Drawing for the job (mm, zero at the part's lowest x, y, z). Give positions to 0.01 mm unless a question says otherwise; leave off trailing zeros. Loops run counter-clockwise (first coordinate to the right, second up) from the corner with the lowest first, then second, coordinate; pieces in that order, holes last. Notation, with made-up numbers: (-11.75, 61) -> (10.25, 61) arc R20 ccw to (10.25, 74) -> close; hole circle Ø3 at (9.5, 86). An arc over 180 degrees is marked (long way). Write item = value, one per line.
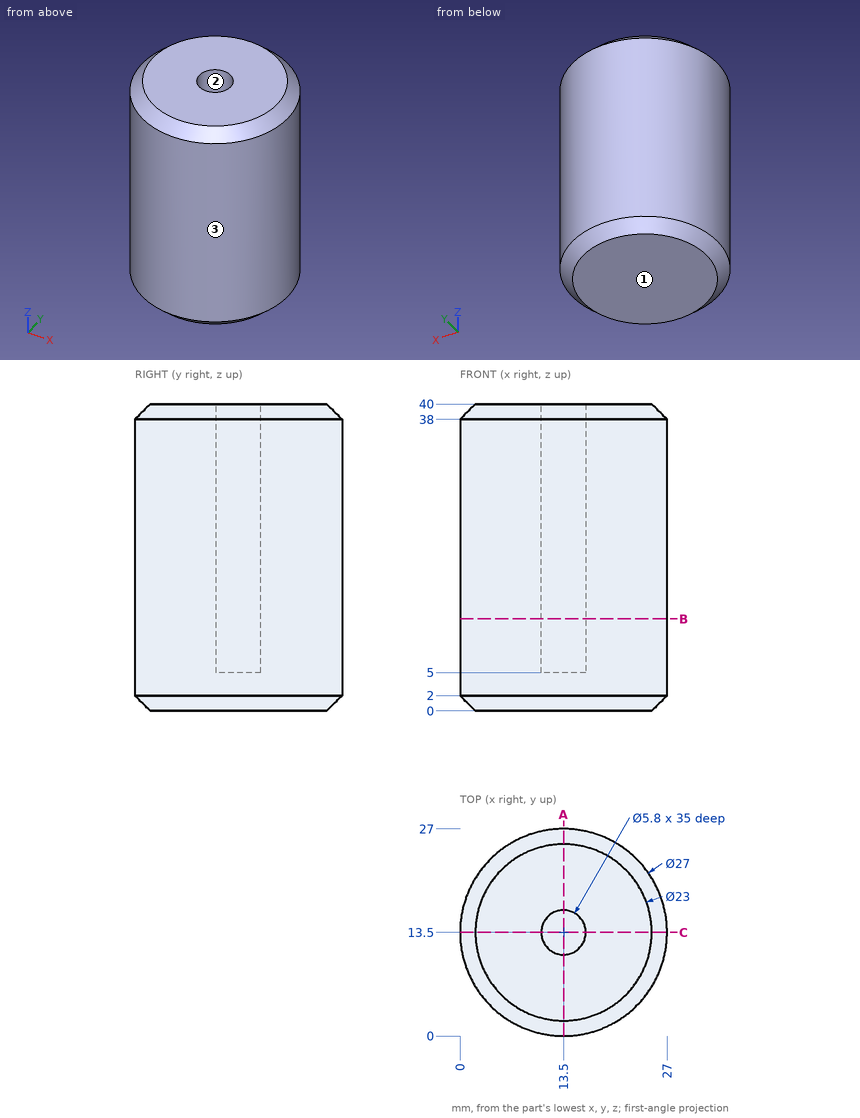
1) Slice it at B-B, the plane z = 12. List the corners of the cut face in (x, y).
Resolved:
outline = circle Ø27 at (13.5, 13.5); hole circle Ø5.8 at (13.5, 13.5)
2) Drop flat-ended pins along their axis: P1, Ø5, axis at x = 13.5, y = 13.5, coming from the +Z side; P2, Ø2, axis at x = 21.5, z = 21.5, coming from the -Y side; P3, Ø12, axis at x = 21, z = 24, coming from the +Y side. Give the stop position or say it passes through.
Resolved:
P1 = 5
P2 = 1.96
P3 = 26.92
3) Pull direction X, two halves, no side cores. Call the marked faces 1, 2 and 3: pulls with the +X half, pulls with the -X half, needs draft (parallel to the pull), parting line crosses it, or undercut.
Resolved:
face_1 = needs draft
face_2 = undercut
face_3 = parting line crosses it
4) Drill centre lines: line 1 along Y through (x, z) = (13.5, 14.5); line 2 along Z through (x, y) = (15, 13.75); line 3 along Z through (x, y) = (13.5, 2). Where is each one in solid material? Low to high. Write a range as [from, to].
Resolved:
line_1 = [0, 10.6], [16.4, 27]
line_2 = [0, 5]
line_3 = [0, 40]
5) Slice it at A-A, the plane x = 13.5. List the corners of the cut face in (y, z), and give its area (3 significant figures).
Resolved:
outline = (0, 2) -> (2, 0) -> (25, 0) -> (27, 2) -> (27, 38) -> (25, 40) -> (16.4, 40) -> (16.4, 5) -> (10.6, 5) -> (10.6, 40) -> (2, 40) -> (0, 38) -> close
area = 869 mm²
